Autodesk Inventor part; units mm, degrees
ref_plane "YZ Plane" through (0, 0, 0) normal (1, 0, 0) x (0, 1, 0)
ref_plane "XZ Plane" through (0, 0, 0) normal (0, 1, 0) x (-1, 0, 0)
ref_plane "XY Plane" through (0, 0, 0) normal (0, 0, 1) x (1, 0, 0)
sketch "Sketch1" plane through (0, 0, 0) normal (0, 0, 1) x (1, 0, 0)
  line L0 (-6.1, 11.1) -> (6.1, 11.1)
  line L1 (7.1, 10.1) -> (7.1, -10.1)
  line L2 (6.1, -11.1) -> (-6.1, -11.1)
  line L3 (-7.1, -10.1) -> (-7.1, 10.1)
  arc A0 (-7.1, -10.1) -> (-6.1, -11.1) centre (-6.1, -10.1) ccw
  arc A1 (6.1, -11.1) -> (7.1, -10.1) centre (6.1, -10.1) ccw
  arc A2 (7.1, 10.1) -> (6.1, 11.1) centre (6.1, 10.1) ccw
  arc A3 (-6.1, 11.1) -> (-7.1, 10.1) centre (-6.1, 10.1) ccw
  circle A4 centre (-12, 0) radius 1.7
  circle A5 centre (-12, -9) radius 1.7
  circle A6 centre (12, 0) radius 1.7
  circle A7 centre (12, -9) radius 1.7
  line L4 (-12, 13.1) -> (6.6, 13.1)
  line L5 (15, 2.7) -> (15, -10.1)
  line L6 (12, -13.1) -> (-12, -13.1)
  line L7 (-15, -10.1) -> (-15, 10.1)
  arc A8 (-12, 13.1) -> (-15, 10.1) centre (-12, 10.1) ccw
  arc A9 (15, 10.1) -> (12, 13.1) centre (12, 10.1) ccw
  arc A10 (12, -13.1) -> (15, -10.1) centre (12, -10.1) ccw
  arc A11 (-15, -10.1) -> (-12, -13.1) centre (-12, -10.1) ccw
  line L8 (8.6, 13.1) -> (15, 13.1)
  line L9 (15, 13.1) -> (15, 4.7)
  line L10 (13, 4.7) -> (11.6, 4.7)
  line L11 (8.6, 7.7) -> (8.6, 11.1)
  arc A12 (8.6, 7.7) -> (11.6, 4.7) centre (11.6, 7.7) ccw
  arc A13 (8.6, 11.1) -> (6.6, 13.1) centre (6.6, 11.1) ccw
  arc A14 (15, 2.7) -> (13, 4.7) centre (13, 2.7) ccw
  line L12 (0, 11.1) -> (0, -11.1) construction
  line L13 (-13, 4.7) -> (-11.6, 4.7)
  line L14 (-8.6, 7.7) -> (-8.6, 11.1)
  arc A15 (-11.6, 4.7) -> (-8.6, 7.7) centre (-11.6, 7.7) ccw
  arc A16 (-6.6, 13.1) -> (-8.6, 11.1) centre (-6.6, 11.1) ccw
  arc A17 (-13, 4.7) -> (-15, 2.7) centre (-13, 2.7) ccw
  point P0 (0, 0)
  point P1 (7.1, -11.1)
  point P2 (7.1, 11.1)
  point P3 (-7.1, -11.1)
  point P4 (-6.6, 13.1)
  dimension "d0" = 14.2
  dimension "d1" = 22.2
  dimension "d2" = 1
  dimension "d3" = 7.1
  dimension "d4" = 11.1
  dimension "d5" = 3.4
  dimension "d8" = 9
  dimension "d11" = 24
  dimension "d14" = 0
  dimension "d15" = 12
  dimension "d16" = 3
  dimension "d17" = 3
  dimension "d18" = 2
  dimension "d19" = 2
  dimension "d20" = 3
  dimension "d23" = 1.5
  dimension "d24" = 3
  dimension "d25" = 3
  dimension "d26" = 2
extrude "Extrusion1" add sketch "Sketch1" along normal blind 3 contours L4 A13 L11 A12 L10 A14 L5 A10 L6 A11 L7 A17 L13 A15 L14 A16
equation "\"d17\" = d16"
properties part number "skye_airspeed_inside_back"
Work out the finished part from the listing and answer in its coordinate system (mm). A direction names the side the tool comes from. Give positions to 0.01 mm unless a question says otherwise; leave off trailing zeros. Write each loop counter-clockwise with the first axis right and the second up, starting at its lowest first coordinate (ties: lowest second). Pieces come first, ordered by that corner, then holes.
(1) The part is cut by section C-C on x = -2. Write down the section's boundary in (y, z).
Final values:
outline: (-13.1, 0) - (-11.1, 0) - (-11.1, 3) - (-13.1, 3) - close; (11.1, 0) - (13.1, 0) - (13.1, 3) - (11.1, 3) - close
(2) The part is cut by section B-B on y = 0. Write down the section's boundary in (x, z).
Final values:
outline: (-15, 0) - (-13.7, 0) - (-13.7, 3) - (-15, 3) - close; (-10.3, 0) - (-7.1, 0) - (-7.1, 3) - (-10.3, 3) - close; (7.1, 0) - (10.3, 0) - (10.3, 3) - (7.1, 3) - close; (13.7, 0) - (15, 0) - (15, 3) - (13.7, 3) - close
(3) Which of the six approach directions +Z, -Z, +X, -X, +Y, -Y give full straight-line access (tool end or side, diameter ignored) to faces 1 (the flat face through (0, 11.1, 1)), 2 (the flat face through (12, 4.7, 1)), 3 (the flat face through (-12, 4.7, 1))?
Final values:
face 1: +Z, -Z
face 2: +Z, -Z, +X, +Y
face 3: +Z, -Z, -X, +Y
(4) The mould has two halves that part along X. Classify faces 4 (the cylindrical face through (-14.43, 4.1, 1.48)), 5 (the flat face through (-7.1, 0, 1)), 6 (the flat face through (-0.2, -11.5, 0)): pulls with the +X half, pulls with the -X half, needs draft (parallel to the pull), parting line crosses it, or undercut.
Final values:
face 4: pulls with the -X half
face 5: undercut
face 6: needs draft
(5) The part is cut by section A-A on y = -5. Write down the section's boundary in (x, z), plus the area to 3 significant figures.
Final values:
outline: (-15, 0) - (-7.1, 0) - (-7.1, 3) - (-15, 3) - close; (7.1, 0) - (15, 0) - (15, 3) - (7.1, 3) - close
area: 47.4 mm2
(6) A flat-ended cylindrical pin translates along its axis: pin 1 Ø2.5 at (x, y) = (-12, 0) entering from +Z. Find the tip coordinate at first contact, or state that the pin passes through.
Final values:
pin 1: passes through
(7) The part is cut by section D-D on z = 2.5. Write down the section's boundary in (x, y), plus the area to 3 significant figures.
Final values:
outline: (-15, -10.1) arc R3 ccw to (-12, -13.1) - (12, -13.1) arc R3 ccw to (15, -10.1) - (15, 2.7) arc R2 ccw to (13, 4.7) - (11.6, 4.7) arc R3 cw to (8.6, 7.7) - (8.6, 11.1) arc R2 ccw to (6.6, 13.1) - (-6.6, 13.1) arc R2 ccw to (-8.6, 11.1) - (-8.6, 7.7) arc R3 cw to (-11.6, 4.7) - (-13, 4.7) arc R2 ccw to (-15, 2.7) - close; hole circle Ø3.4 at (-12, -9); hole circle Ø3.4 at (-12, 0); hole (-7.1, -10.1) arc R1 ccw to (-6.1, -11.1) - (6.1, -11.1) arc R1 ccw to (7.1, -10.1) - (7.1, 10.1) arc R1 ccw to (6.1, 11.1) - (-6.1, 11.1) arc R1 ccw to (-7.1, 10.1) - close; hole circle Ø3.4 at (12, -9); hole circle Ø3.4 at (12, 0)
area: 324 mm2
(8) Straight lines are drawn through the part: line 1 (Y direction, x = -12, z = 1.15); line 2 (Y direction, x = -1.25, z = 1); line 3 (X direction, y = -9.25, z = 2.6). For each, find the intervals that lie inside material, in ascending order.
Final values:
line 1: y = -13.1 to -10.7, -7.3 to -1.7, 1.7 to 4.7
line 2: y = -13.1 to -11.1, 11.1 to 13.1
line 3: x = -15 to -13.68, -10.32 to -7.1, 7.1 to 10.32, 13.68 to 15
